from build123d import *

# Parameters (mm, degrees)
F0_R     = 10
F1_DEPTH = 20
F3_R     = 5.08
F4_DEPTH = 25
F5_DEPTH = 25.4
F6_R     = 7.75
F7_DEPTH = 16
F8_R     = 2.5
F9_DEPTH = 3


with BuildPart() as f1:
    # F0 (on Top) → F1 (new body)
    with BuildSketch(Plane.XY):
        Circle(F0_R)
    extrude(amount=F1_DEPTH)

    # F3
    f3_edges = [f1.edges().sort_by_distance(p)[0] for p in [
        (-10, 0, 20),
    ]]
    fillet(f3_edges, radius=F3_R)

    # F2 (on Front) → F4 (cut)
    with BuildSketch(Plane.XZ):
        with BuildLine():
            Line((13.2011724636, 2.0541311242), (10.8197718092, 13.8740318547))
            Line((10.8197718092, 13.8740318547), (2.8975781604, 12.7609964594))
            ThreePointArc((2.8975781604, 12.7609964594), (1.666446785, 12.0925993918), (1.1758370092, 10.7804480472))
            Line((1.1758370092, 10.7804480472), (1.1758370092, 5.7804480472))
            ThreePointArc((1.1758370092, 5.7804480472), (1.6481085109, 4.4896941453), (2.8418826446, 3.8085265269))
            Line((2.8418826446, 3.8085265269), (13.2011724636, 2.0541311242))
        make_face()
    extrude(amount=-F4_DEPTH, mode=Mode.SUBTRACT)

    # F5 (cut): a face of the model
    f5_faces = [f1.faces().sort_by_distance(p)[0] for p in [
        (5.8523701774, 0, 8.2355862053),
    ]]
    extrude(f5_faces, amount=-F5_DEPTH, mode=Mode.SUBTRACT)

    # F6 (on face) → F7 (cut)
    with BuildSketch(Plane(origin=(0, 0, 0), x_dir=(1, 0, 0), z_dir=(0, 0, -1))):
        Circle(F6_R)
    extrude(amount=-F7_DEPTH, mode=Mode.SUBTRACT)

    # F8 (on face) → F9 (cut)
    with BuildSketch(Plane(origin=(0, 0, 16), x_dir=(1, 0, 0), z_dir=(0, 0, -1))):
        Circle(F8_R)
    extrude(amount=-F9_DEPTH, mode=Mode.SUBTRACT)


solid = f1.part
The listing builds one solid part. Answer for the finished solid, in the listing's coordinates (mm). A direction names the side the tool comes from. Coordinates: 2 decimals unless noted, no trailing zeros. Loops run counter-clockwise (first coordinate to the right, second up) from the corner with the lowest first, then second, coordinate; pieces in that order, holes last. Notation, with made-up numbers: (-7, -2) -> (11, -2) arc R15 cw to (11, 16) -> close; hole circle Ø2 at (87, -17). An arc over 180 degrees is marked (long way). Answer in a Markdown table with one row per item. Add a question column.
1. Determine the mould class of faces 4 (the flat face through (0, 0, 20)), 5 (the cylindrical face through (1.68, -8.54, 12.11)), 6 (the cylindrical face through (-0.54, 2.44, 17.48)) for opening direction Z: +Z half, -Z half, draft (parallel to the pull), parting line (faces both ways), or undercut.
2. Flat-ended cylindrical pins translate along their axes: P1, Ø8, axis at x = -1, y = -3, coming from the -Z side; P2, Ø3, axis at x = -2, z = 13, coming from the -Y side; P3, Ø2.5, axis at y = 9, z = 8.5, coming from the +X side. Find the tip coordinate at first contact, or state that the pin passes through.
3. The part is cut by section A-A, the plane z = 3.5. Write down the section's boundary in (x, y), then the cut area to 3 significant figures.
4. Consider line 1 (Y direction, x = 0, z = 11); line 2 (Z direction, x = 4.5, y = 1.5); line 3 (X direction, y = 0, z = 17). Determine where each line is inside the solid, lowest interval first. Write a range as [from, to].
5. For faces 1 (the flat face through (0, 0, 19)), 2 (the cylindrical face through (-10, 0, 7)), 3 (the flat face through (1.176, -9, 8)), determine the directions among +Z, -Z, +X, -X, +Y, -Y from which every point of the face is accessible in a straight line to the end or side of a thin tool.
Answer below:
| question | item | result |
|---|---|---|
| 1 | face 4 | +Z half |
| 1 | face 5 | undercut |
| 1 | face 6 | draft |
| 2 | P1 | z = 16 |
| 2 | P2 | y = -9.99 |
| 2 | P3 | x = 1.18 |
| 3 | outline | (4.66, -8.85) -> (4.66, -6.19) arc R7.75 cw (long way) to (4.66, 6.19) -> (4.66, 8.85) arc R10 ccw (long way) to start |
| 3 | area | 84.9 mm2 |
| 4 | line 1 | [-10, -7.75], [7.75, 10] |
| 4 | line 2 | [16, 20] |
| 4 | line 3 | [-9.55, -2.5], [2.5, 9.55] |
| 5 | face 1 | -Z |
| 5 | face 2 | +Z, -Z |
| 5 | face 3 | +X, +Y, -Y |
